Can you work these out from the model? Positions are in its coordinate system, mm. A direction names the side the tool comes from. Coordinates: 2 decimals unless noted, no trailing zeros. Write each loop counter-clockwise with the first axis right and the second up, starting at its lowest first coordinate (ties: lowest second). Pieces come first, ordered by that corner, then holes. Notation, with made-up numbers: M -33,84 L 5,84 A23 ccw 5,102 Z; hole C 43,24 d10. An arc over 180 degrees is marked long. Use one line per item in the form item = value. Start each with the question number.
```python
from build123d import *

# Parameters (mm, degrees)
SKETCH1_R           = 2.5
BOSS_EXTRUDE3_DEPTH = 3
SKETCH4_R           = 4
SKETCH4_R_2         = 2.5
BOSS_EXTRUDE4_DEPTH = 3
FILLET1_R           = 1
FILLET2_R           = 0.25


with BuildPart() as part:
    # Sketch1 → Boss-Extrude3 (new body)
    with BuildSketch(Plane.XY):
        with BuildLine():
            Line((-0.612376666, 7.250336436), (-0.775314301, 6.33381714))
            ThreePointArc((-0.775314301, 6.33381714), (-1.244889549, 6.258482391), (-1.707549869, 6.148383956))
            Line((-1.707549869, 6.148383956), (-2.208821365, 6.932783841))
            Line((-2.208821365, 6.932783841), (-2.682669744, 7.403979203))
            Line((-2.682669744, 7.403979203), (-3.01363203, 7.275551319))
            Line((-3.01363203, 7.275551319), (-3.338469935, 7.13233787))
            Line((-3.338469935, 7.13233787), (-3.340345901, 6.464091033))
            Line((-3.340345901, 6.464091033), (-3.140143897, 5.554984081))
            ThreePointArc((-3.140143897, 5.554984081), (-3.545145497, 5.30568518), (-3.930455051, 5.02691505))
            Line((-3.930455051, 5.02691505), (-4.693746367, 5.559777753))
            Line((-4.693746367, 5.559777753), (-5.311843844, 5.813771579))
            Line((-5.311843844, 5.813771579), (-5.568465902, 5.568465902))
            Line((-5.568465902, 5.568465902), (-5.813771579, 5.311843844))
            Line((-5.813771579, 5.311843844), (-5.559777753, 4.693746367))
            Line((-5.559777753, 4.693746367), (-5.02691505, 3.930455051))
            ThreePointArc((-5.02691505, 3.930455051), (-5.30568518, 3.545145497), (-5.554984081, 3.140143897))
            Line((-5.554984081, 3.140143897), (-6.464091033, 3.340345901))
            Line((-6.464091033, 3.340345901), (-7.13233787, 3.338469935))
            Line((-7.13233787, 3.338469935), (-7.275551319, 3.01363203))
            Line((-7.275551319, 3.01363203), (-7.403979203, 2.682669744))
            Line((-7.403979203, 2.682669744), (-6.932783841, 2.208821365))
            Line((-6.932783841, 2.208821365), (-6.148383956, 1.707549869))
            ThreePointArc((-6.148383956, 1.707549869), (-6.258482391, 1.244889549), (-6.33381714, 0.775314301))
            Line((-6.33381714, 0.775314301), (-7.250336436, 0.612376666))
            Line((-7.250336436, 0.612376666), (-7.866998111, 0.354916505))
            Line((-7.866998111, 0.354916505), (-7.875, 0))
            Line((-7.875, 0), (-7.866998111, -0.354916505))
            Line((-7.866998111, -0.354916505), (-7.250336436, -0.612376666))
            Line((-7.250336436, -0.612376666), (-6.33381714, -0.775314301))
            ThreePointArc((-6.33381714, -0.775314301), (-6.258482391, -1.244889549), (-6.148383956, -1.707549869))
            Line((-6.148383956, -1.707549869), (-6.932783841, -2.208821365))
            Line((-6.932783841, -2.208821365), (-7.403979203, -2.682669744))
            Line((-7.403979203, -2.682669744), (-7.275551319, -3.01363203))
            Line((-7.275551319, -3.01363203), (-7.13233787, -3.338469935))
            Line((-7.13233787, -3.338469935), (-6.464091033, -3.340345901))
            Line((-6.464091033, -3.340345901), (-5.554984081, -3.140143897))
            ThreePointArc((-5.554984081, -3.140143897), (-5.30568518, -3.545145497), (-5.02691505, -3.930455051))
            Line((-5.02691505, -3.930455051), (-5.559777753, -4.693746367))
            Line((-5.559777753, -4.693746367), (-5.813771579, -5.311843844))
            Line((-5.813771579, -5.311843844), (-5.568465902, -5.568465902))
            Line((-5.568465902, -5.568465902), (-5.311843844, -5.813771579))
            Line((-5.311843844, -5.813771579), (-4.693746367, -5.559777753))
            Line((-4.693746367, -5.559777753), (-3.930455051, -5.02691505))
            ThreePointArc((-3.930455051, -5.02691505), (-3.545145497, -5.30568518), (-3.140143897, -5.554984081))
            Line((-3.140143897, -5.554984081), (-3.340345901, -6.464091033))
            Line((-3.340345901, -6.464091033), (-3.338469935, -7.13233787))
            Line((-3.338469935, -7.13233787), (-3.01363203, -7.275551319))
            Line((-3.01363203, -7.275551319), (-2.682669744, -7.403979203))
            Line((-2.682669744, -7.403979203), (-2.208821365, -6.932783841))
            Line((-2.208821365, -6.932783841), (-1.707549869, -6.148383956))
            ThreePointArc((-1.707549869, -6.148383956), (-1.244889549, -6.258482391), (-0.775314301, -6.33381714))
            Line((-0.775314301, -6.33381714), (-0.612376666, -7.250336436))
            Line((-0.612376666, -7.250336436), (-0.354916505, -7.866998111))
            Line((-0.354916505, -7.866998111), (0, -7.875))
            Line((0, -7.875), (0.354916505, -7.866998111))
            Line((0.354916505, -7.866998111), (0.612376666, -7.250336436))
            Line((0.612376666, -7.250336436), (0.775314301, -6.33381714))
            ThreePointArc((0.775314301, -6.33381714), (1.244889549, -6.258482391), (1.707549869, -6.148383956))
            Line((1.707549869, -6.148383956), (2.208821365, -6.932783841))
            Line((2.208821365, -6.932783841), (2.682669744, -7.403979203))
            Line((2.682669744, -7.403979203), (3.01363203, -7.275551319))
            Line((3.01363203, -7.275551319), (3.338469935, -7.13233787))
            Line((3.338469935, -7.13233787), (3.340345901, -6.464091033))
            Line((3.340345901, -6.464091033), (3.140143897, -5.554984081))
            ThreePointArc((3.140143897, -5.554984081), (3.545145497, -5.30568518), (3.930455051, -5.02691505))
            Line((3.930455051, -5.02691505), (4.693746367, -5.559777753))
            Line((4.693746367, -5.559777753), (5.311843844, -5.813771579))
            Line((5.311843844, -5.813771579), (5.568465902, -5.568465902))
            Line((5.568465902, -5.568465902), (5.813771579, -5.311843844))
            Line((5.813771579, -5.311843844), (5.559777753, -4.693746367))
            Line((5.559777753, -4.693746367), (5.02691505, -3.930455051))
            ThreePointArc((5.02691505, -3.930455051), (5.30568518, -3.545145497), (5.554984081, -3.140143897))
            Line((5.554984081, -3.140143897), (6.464091033, -3.340345901))
            Line((6.464091033, -3.340345901), (7.13233787, -3.338469935))
            Line((7.13233787, -3.338469935), (7.275551319, -3.01363203))
            Line((7.275551319, -3.01363203), (7.403979203, -2.682669744))
            Line((7.403979203, -2.682669744), (6.932783841, -2.208821365))
            Line((6.932783841, -2.208821365), (6.148383956, -1.707549869))
            ThreePointArc((6.148383956, -1.707549869), (6.258482391, -1.244889549), (6.33381714, -0.775314301))
            Line((6.33381714, -0.775314301), (7.250336436, -0.612376666))
            Line((7.250336436, -0.612376666), (7.866998111, -0.354916505))
            Line((7.866998111, -0.354916505), (7.875, 0))
            Line((7.875, 0), (7.866998111, 0.354916505))
            Line((7.866998111, 0.354916505), (7.250336436, 0.612376666))
            Line((7.250336436, 0.612376666), (6.33381714, 0.775314301))
            ThreePointArc((6.33381714, 0.775314301), (6.258482391, 1.244889549), (6.148383956, 1.707549869))
            Line((6.148383956, 1.707549869), (6.932783841, 2.208821365))
            Line((6.932783841, 2.208821365), (7.403979203, 2.682669744))
            Line((7.403979203, 2.682669744), (7.275551319, 3.01363203))
            Line((7.275551319, 3.01363203), (7.13233787, 3.338469935))
            Line((7.13233787, 3.338469935), (6.464091033, 3.340345901))
            Line((6.464091033, 3.340345901), (5.554984081, 3.140143897))
            ThreePointArc((5.554984081, 3.140143897), (5.30568518, 3.545145497), (5.02691505, 3.930455051))
            Line((5.02691505, 3.930455051), (5.559777753, 4.693746367))
            Line((5.559777753, 4.693746367), (5.813771579, 5.311843844))
            Line((5.813771579, 5.311843844), (5.568465902, 5.568465902))
            Line((5.568465902, 5.568465902), (5.311843844, 5.813771579))
            Line((5.311843844, 5.813771579), (4.693746367, 5.559777753))
            Line((4.693746367, 5.559777753), (3.930455051, 5.02691505))
            ThreePointArc((3.930455051, 5.02691505), (3.545145497, 5.30568518), (3.140143897, 5.554984081))
            Line((3.140143897, 5.554984081), (3.340345901, 6.464091033))
            Line((3.340345901, 6.464091033), (3.338469935, 7.13233787))
            Line((3.338469935, 7.13233787), (3.01363203, 7.275551319))
            Line((3.01363203, 7.275551319), (2.682669744, 7.403979203))
            Line((2.682669744, 7.403979203), (2.208821365, 6.932783841))
            Line((2.208821365, 6.932783841), (1.707549869, 6.148383956))
            ThreePointArc((1.707549869, 6.148383956), (1.244889549, 6.258482391), (0.775314301, 6.33381714))
            Line((0.775314301, 6.33381714), (0.612376666, 7.250336436))
            Line((0.612376666, 7.250336436), (0.354916505, 7.866998111))
            Line((0.354916505, 7.866998111), (0, 7.875))
            Line((0, 7.875), (-0.354916505, 7.866998111))
            Line((-0.354916505, 7.866998111), (-0.612376666, 7.250336436))
        make_face()
        Circle(SKETCH1_R, mode=Mode.SUBTRACT)
    extrude(amount=BOSS_EXTRUDE3_DEPTH)

    # Sketch4 → Boss-Extrude4 (add)
    with BuildSketch(Plane.XY.offset(3)):
        Circle(SKETCH4_R)
        Circle(SKETCH4_R_2, mode=Mode.SUBTRACT)
    extrude(amount=BOSS_EXTRUDE4_DEPTH)

    # Fillet1
    fillet1_edges = [part.edges().sort_by_distance(p)[0] for p in [
        (-4, 0, 6),
    ]]
    fillet(fillet1_edges, radius=FILLET1_R)

    # Fillet2
    fillet2_edges = [part.edges().sort_by_distance(p)[0] for p in [
        (-2.5, 0, 0),
    ]]
    fillet(fillet2_edges, radius=FILLET2_R)


solid = part.part
```
1) Which directions (+Z, -Z, +X, -X, +Y, -Y) give clear straight access to the entire face, cutting with the end or side of a thin tool? Please do faces 1 (the face through (-3.24, -6, 1.48)), 2 (the face through (0.693, -6.798, 1.479)), 3 (the face through (6.786, -0.695, 1.479)), 4 (the face through (-2, 2, 6)), 5 (the face through (-6.26, -1.24, 1.48)).
2) Suppose I cut it at B-B on y = -4.5. Please give me the cut outline in (x, z).
3) Please list where these lines run through material, in increasing order: line 1 (Y direction, x = 0, z = 4.8); line 2 (Y direction, x = 0, z = 2.75) (3 decimals); line 3 (X direction, y = 6.75, z = 1.45).
4) If we mould it in two halves opening along Y, with no side actions, what happens to faces 6 (the face through (-0.693, 6.798, 1.479)), 7 (the face through (3, 0, 0)), 8 (the face through (6.016, 3.242, 1.479)), 9 (the face through (-6.798, -0.693, 1.479))? For each: +Y half, -Y half, draft (parallel to the pull), parting line (faces both ways), or undercut.
5) Will these pins go through, and if not, where does the flat tip stop? pin 1 Ø2 at (x, z) = (2, 1.5) entering from -Y; pin 2 Ø1 at (x, y) = (-3.5, -4) entering from +Z.
6) Suppose I cut it at A-A on z = 3.9. Please give me the cut outline in (x, y), and give its area (3 significant figures).
Computed values:
q1.face_1 = +Z, -Z
q1.face_2 = +Z, -Z, -Y
q1.face_3 = +Z, -Z, +X
q1.face_4 = +Z, +X, -X, +Y, -Y
q1.face_5 = +Z, -Z, -X
q2.outline = M -5.42,0 L 5.42,0 L 5.42,3 L -5.42,3 Z
q3.line_1 = -4 to -2.5, 2.5 to 4
q3.line_2 = -7.875 to -2.5, 2.5 to 7.875
q3.line_3 = -3.34 to -2.09, -0.7 to 0.7, 2.09 to 3.34
q4.face_6 = +Y half
q4.face_7 = draft
q4.face_8 = undercut
q4.face_9 = undercut
q5.pin_1 = -7.4
q5.pin_2 = 3
q6.outline = C 0,0 d8; hole C 0,0 d5
q6.area = 30.6 mm²
